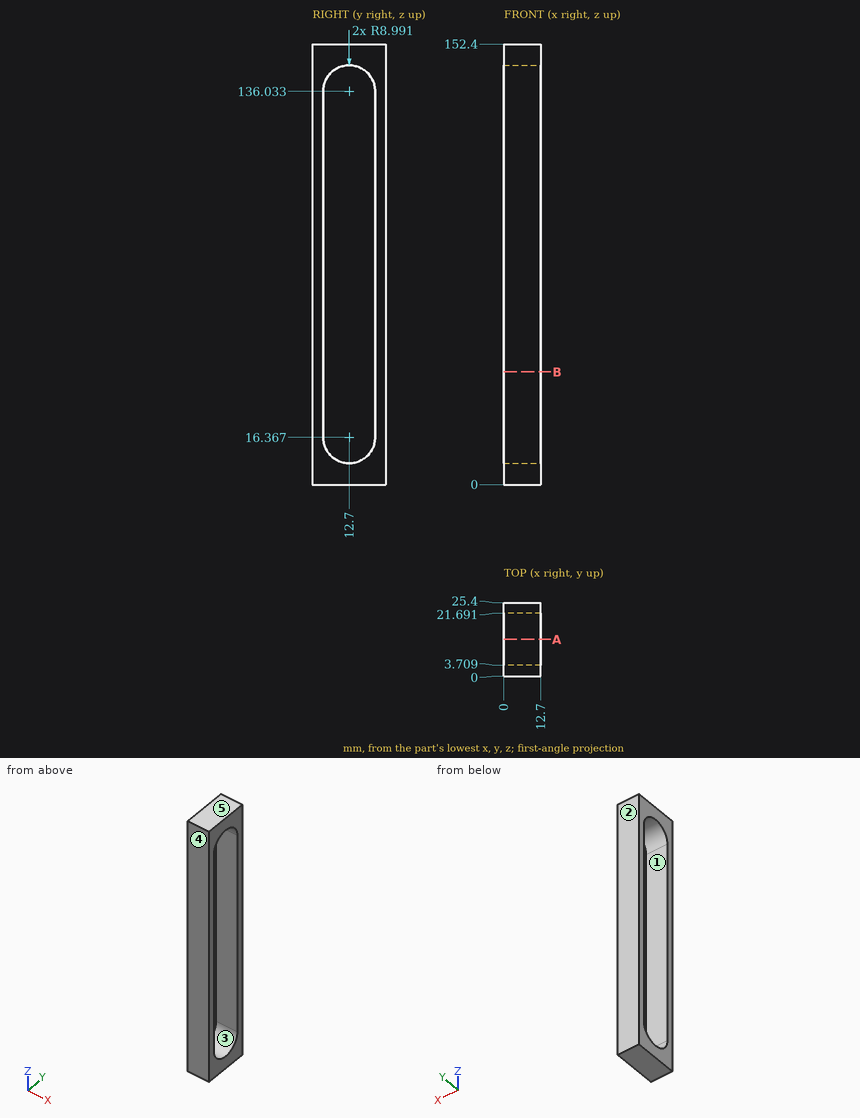
Here's the drawing with two shaded views (mm, measured from the low corner). I have some questions. A direction names the side the tool comes from. Give positions to 0.01 mm unless a question says otherwise; leave off trailing zeros. Order: outer loops, then holes, each group sorted by start corner. A loop starts at its lowest first (then second) coordinate and runs counter-clockwise, first axis right, second up. Notation, with made-up numbers: (20.5, -35) -> (28.5, -35) arc R8 cw to (28.5, -31) -> close; hole circle Ø5 at (63.25, 6). An arc over 180 degrees is marked (long way). Use a Markdown table: item, result. Add a question column.
Item 1: Imagine slicing it at B-B on z = 39. Please give me the cut outline in (x, y).
Item 2: Will this pin go through, and if not, where does the flat tip stop? pin 1 (2 mm diameter, centred on y = 3.5, z = 83.5, fed in from -X).
Item 3: For the marked faces 1 and 2, which set-ups out of +Z, -Z, +X, -X, +Y, -Y let a thin tool reach every point of the face, with its end or its side?
Item 4: I need wall thicknesses on line 1 (Y direction, x = 8.5, z = 111); line 2 (Z direction, x = 11.25, y = 13); line 3 (Z direction, x = 4.75, y = 18.25) (1 decimal). Which ranges of each line are inside material? Lowest first, please.
Item 5: If we mould it in two halves opening along Z, with no side actions, what happens to the marked faces 3, 4 and 5? For each: pulls with the +Z half, pulls with the -Z half, needs draft (parallel to the pull), parting line crosses it, or undercut.
Item 6: Imagine slicing it at A-A on y = 12.7. Please give me the cut outline in (x, z) (1 decimal).
Data:
| question | item | result |
|---|---|---|
| 1 | outline | (0, 0) -> (12.7, 0) -> (12.7, 3.71) -> (0, 3.71) -> close; (0, 21.69) -> (12.7, 21.69) -> (12.7, 25.4) -> (0, 25.4) -> close |
| 2 | pin 1 | stops at x = 0 |
| 3 | face 1 | +X, -X |
| 3 | face 2 | +Z, -Z, +X, -X, +Y |
| 4 | line 1 | y = 0 to 3.71, 21.69 to 25.4 |
| 4 | line 2 | z = 0 to 7.38, 145.02 to 152.4 |
| 4 | line 3 | z = 0 to 9.3, 143.1 to 152.4 |
| 5 | face 3 | undercut |
| 5 | face 4 | needs draft |
| 5 | face 5 | pulls with the +Z half |
| 6 | outline | (0, 0) -> (12.7, 0) -> (12.7, 7.4) -> (0, 7.4) -> close; (0, 145) -> (12.7, 145) -> (12.7, 152.4) -> (0, 152.4) -> close |
